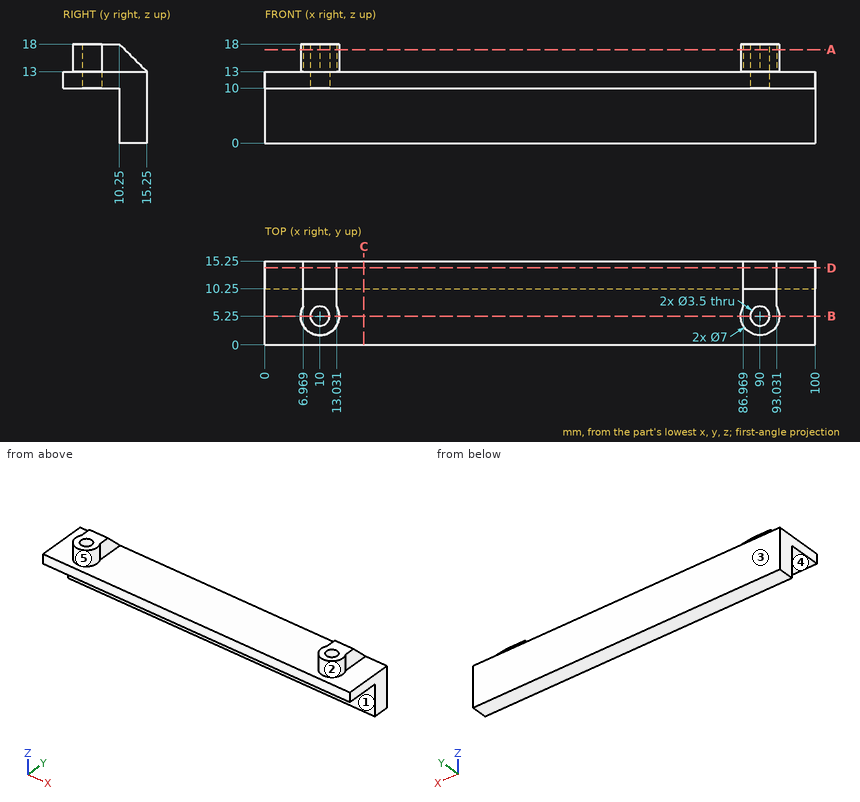
Geometry check sheet. Reference: drawing and pictorial views, mm from the part's lowest x, y, z. A direction names the side the tool comes from. Round coordinates to 2 decimals unless told otherwise and drop trailing zeros. Loops run counter-clockwise (first coordinate to the right, second up) from the corner with the lowest first, then second, coordinate; pieces in that order, holes last. Notation, with made-up numbers: (16, -38.75) - (54, -38.75) arc R9 cw to (54, -22.75) - close; hole circle Ø10 at (-0.75, -9). An arc over 180 degrees is marked (long way). Use a Markdown table: item, result. Add a question column.
1. Section check A-A, the plane z = 17. Record the boundary of the cut face in (x, y).
2. Access from +Z, -Z, +X, -X, +Y, -Y to the whole of each face (thin tool, end or side, straight path). Record for the marked faces 3, 4 and 5.
3. Section check B-B, the plane y = 5.25. Record the boundary of the cut face in (x, z), plus the area to 3 significant figures.
4. Gauge pin test, flat ends, axial feed: pin 1 (4 mm diameter, centred on x = 90, y = 5.25, fed in from +Z); pin 2 (3 mm diameter, centred on x = 10, y = 5.25, fed in from -Z); pin 3 (8 mm diameter, centred on x = 60.5, z = 5, fed in from -Y). Record the tip position at first contact, or that the pin passes through.
5. Release check for a two-part mould opening along X. For the marked faces 1 and 2 record: released by +X, released by -X, zero draft, split by the parting line, or undercut.
6. Section check D-D, the plane y = 14. Record the boundary of the cut face in (x, z), plus the area to 3 significant figures.
7. Thickness scan on probe 1 along X at (y, z) = (5.25, 13.25); probe 2 along X at (y, z) = (8.25, 13.5); probe 3 along Y at (x, z) = (90, 15.5). Record the ranges inside material, lowest first. Write a range as [from, to].
8. Section check C-C, the plane x = 18. Record the boundary of the cut face in (y, z).
Checks:
| question | item | result |
|---|---|---|
| 1 | outline | (6.97, 7) arc R3.5 ccw (long way) to (13.03, 7) - (13.03, 11.25) - (6.97, 11.25) - close; (86.97, 7) arc R3.5 ccw (long way) to (93.03, 7) - (93.03, 11.25) - (86.97, 11.25) - close; hole circle Ø3.5 at (10, 5.25); hole circle Ø3.5 at (90, 5.25) |
| 2 | face 3 | +Z, -Z, +X, -X, +Y |
| 2 | face 4 | -Z, +X, -X, -Y |
| 2 | face 5 | +Z |
| 3 | outline | (0, 10) - (8.25, 10) - (8.25, 18) - (6.5, 18) - (6.5, 13) - (0, 13) - close; (11.75, 10) - (88.25, 10) - (88.25, 18) - (86.5, 18) - (86.5, 13) - (13.5, 13) - (13.5, 18) - (11.75, 18) - close; (91.75, 10) - (100, 10) - (100, 13) - (93.5, 13) - (93.5, 18) - (91.75, 18) - close |
| 3 | area | 314 mm^2 |
| 4 | pin 1 | stops at z = 18 |
| 4 | pin 2 | passes through |
| 4 | pin 3 | stops at y = 10.25 |
| 5 | face 1 | zero draft |
| 5 | face 2 | undercut |
| 6 | outline | (0, 0) - (100, 0) - (100, 13) - (93.03, 13) - (93.03, 14.25) - (86.97, 14.25) - (86.97, 13) - (13.03, 13) - (13.03, 14.25) - (6.97, 14.25) - (6.97, 13) - (0, 13) - close |
| 6 | area | 1,320 mm^2 |
| 7 | probe 1 | x = [6.5, 8.25], [11.75, 13.5], [86.5, 88.25], [91.75, 93.5] |
| 7 | probe 2 | x = [6.97, 13.03], [86.97, 93.03] |
| 7 | probe 3 | y = [1.75, 3.5], [7, 12.75] |
| 8 | outline | (0, 10) - (10.25, 10) - (10.25, 0) - (15.25, 0) - (15.25, 13) - (0, 13) - close |
